Check sheet for the modelled part. Datum: model origin and axes. Units: mm. A direction names the side the tool comes from. Round coordinates to 2 decimals unless told otherwise and drop trailing zeros. Loops run counter-clockwise (first coordinate to the right, second up) from the corner with the lowest first, then second, coordinate; pieces in that order, holes last. Notation, with made-up numbers: M 1.5,50.5 L 9.5,50.5 A11 ccw 9.5,57.5 Z; hole C -2,47 d10. An arc over 180 degrees is marked long. One line per question, with ' | ' between items. Start each with the question number.
(1) Section check C-C (z = -0.5). Record the boundary of the cut face in (x, y), and give its area (3 significant figures).
(2) Go/stop test with flat-tipped pins: P1, Ø1.5, axis at x = -9.5, z = -0.5, coming from the -Y side; P2, Ø2, axis at x = -2.5, z = 4, coming from the -Y side; P3, Ø1.5, axis at x = 2, y = 4.5, coming from the -Z side; P4, Ø8, axis at x = 1, y = -2, coming from the +Z side. Record where each tip stops, or that it passes through.
(3) Section check A-A (y = 0). Record the boundary of the cut face in (x, z).
(4) Section check D-D (y = -10.5). Record the boundary of the cut face in (x, z), and give its area (3 significant figures).
(5) Thickness scan on probe 1 along Y at (x, z) = (0, -5.1); probe 2 along Y at (x, z) = (0, -1.5); probe 3 along X at (y, z) = (-3.5, 1). Record the ranges inside material, lowest first. Write a range as [from, to].
(6) Tool access check on faces 5 (the face through (-3, -5.4, -5.5)), 6 (the face through (-1.73, -7.81, 0.06)). Record the directions out of +Z, -Z, +X, -X, +Y, -Y that give a thin tool (end or side, any length) a straight path to the whole face; none if there is none.
(7) Draft check along Y on faces 1 (the face through (11.923, 3.755, 0.077)), 2 (the face through (-6, 0, -5)), 3 (the face through (-2, 6, -4.5)), 4 (the face through (-9, 3, 5.5)). Enter one of: +Y half, -Y half, draft (parallel to the pull), parting line (faces both ways), or undercut.
Autodesk Inventor part; units mm, degrees
ref_plane "YZ Plane" through (0, 0, 0) normal (1, 0, 0) x (0, 1, 0)
ref_plane "XZ Plane" through (0, 0, 0) normal (0, 1, 0) x (-1, 0, 0)
ref_plane "XY Plane" through (0, 0, 0) normal (0, 0, 1) x (1, 0, 0)
sketch "Szkic główny" plane through (0, 0, 0) normal (0, 0, 1) x (1, 0, 0)
  circle A0 centre (0, 0) radius 12.5
  dimension "d0" = 25
extrude "Koło pasowe" add sketch "Szkic główny" along normal mid plane 11
sketch "Szkic2" plane through (0, 0, 5.5) normal (0, 0, 1) x (1, 0, 0)
  circle A0 centre (0, 0) radius 8
  circle A1 centre (0, 0) radius 6
  dimension "d5" = 16
  dimension "d6" = 12
extrude "Wyciągnięcie proste2" cut sketch "Szkic2" against normal through all contours A1
extrude "Wyciągnięcie proste3" cut sketch "Szkic2" against normal blind 10
chamfer "Faza1" distance 1 angle 45 1 edges at (-8, 0, 5.5)
equation "\"d0\" = da_D"
equation "\"d1\" = da_B"
equation "\"da_D\" = 25"
equation "\"da_B\" = 11"
properties part number "Koło pasowe zwykłe1" material "Steel"
The answers:
1) outline: C 0,0 d25; hole C 0,0 d16 | area: 290 mm²
2) P1: y = -8.93 | P2: y = -12.41 | P3: through | P4: z = -4.5
3) outline: M -12.5,-5.5 L -6,-5.5 L -6,-4.5 L -8,-4.5 L -8,4.5 L -9,5.5 L -12.5,5.5 Z; M 6,-5.5 L 12.5,-5.5 L 12.5,5.5 L 9,5.5 L 8,4.5 L 8,-4.5 L 6,-4.5 Z
4) outline: M -6.78,-5.5 L 6.78,-5.5 L 6.78,5.5 L -6.78,5.5 Z | area: 149 mm²
5) probe 1: [-12.5, -6], [6, 12.5] | probe 2: [-12.5, -8], [8, 12.5] | probe 3: [-12, -7.19], [7.19, 12]
6) face 5: -Z, +X, -X, +Y, -Y | face 6: +Z
7) face 1: parting line | face 2: undercut | face 3: undercut | face 4: draft
